Here's the drawing with two shaded views (mm, measured from the low corner). I have some questions. Coordinates: 2 decimals unless noted, no trailing zeros. Loops run counter-clockwise (first coordinate to the right, second up) from the corner with the lowest first, then second, coordinate; pieces in that order, holes last. Notation, with made-up numbers: (69, 74) - (82, 74) arc R10 ccw to (82, 87) - close; hole circle Ø1 at (-13, 46). An arc over 180 degrees is marked (long way). Use a Markdown table: item, result.
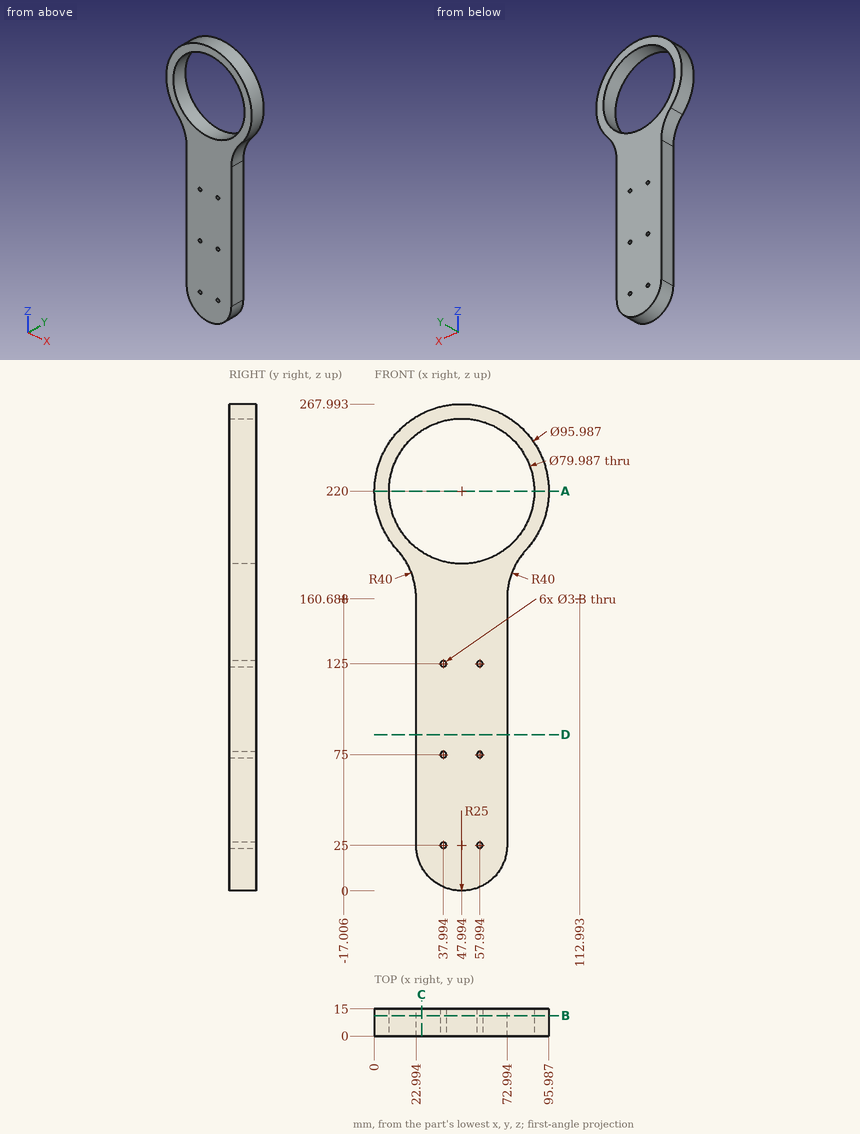
Q1. I want a section at C-C, the plane x = 26. Write out the boundary of the cut face in (y, z).
Check values:
| item | result |
|---|---|
| outline | (0, 13.11) - (15, 13.11) - (15, 186.6) - (0, 186.6) - close; (0, 253.4) - (15, 253.4) - (15, 262.66) - (0, 262.66) - close |
Q2. I want a section at D-D, the plane z = 86. Write out the boundary of the cut face in (x, y), then the cut area to 3 significant figures.
Check values:
| item | result |
|---|---|
| outline | (22.99, 0) - (72.99, 0) - (72.99, 15) - (22.99, 15) - close |
| area | 750 mm^2 |
Q3. I want a section at B-B, the plane y = 11.25. Give the number of separate pieces and of enclosed holes in the cut face, then the cut area to 3 significant figures.
Check values:
| item | result |
|---|---|
| separate pieces | 1 |
| enclosed holes | 7 |
| area | 10,700 mm^2 |
Q4. Will these pins go through, and if not, where does the flat tip stop? P1, Ø4, axis at x = 57.99, z = 25, coming from the +Y side; P2, Ø1, axis at y = 13, z = 76, coming from the -X side; P3, Ø1, axis at y = 10, z = 178.5, coming from the -X side (1 decimal); P4, Ø1.5, axis at x = 29.5, z = 187, coming from the +Y side.
Check values:
| item | result |
|---|---|
| P1 | y = 15 |
| P2 | x = 22.99 |
| P3 | x = 18.6 |
| P4 | through |
Q5. Please list where these lines run through material, in increasing order: L1, parallel to X at y = 9.5, z = 25; L2, parallel to X at y = 2.5, z = 53.5; L3, parallel to Z at x = 11.5, y = 2.5 (1 decimal). Write a range as from..to.
Check values:
| item | result |
|---|---|
| L1 | 22.99..36.34, 39.64..56.34, 59.64..72.99 |
| L2 | 22.99..72.99 |
| L3 | 188.8..203.6, 236.4..251.2 |
Q6. I want a section at A-A, the plane z = 220. Write out the boundary of the cut face in (x, y).
Check values:
| item | result |
|---|---|
| outline | (0, 0) - (8, 0) - (8, 15) - (0, 15) - close; (87.99, 0) - (95.99, 0) - (95.99, 15) - (87.99, 15) - close |
